```python
from build123d import *

# Parameters (mm, degrees)
SKETCH1_R           = 2.8575
BOSS_EXTRUDE1_DEPTH = 3.5052
CUT_EXTRUDE1_DEPTH  = 1.9558
SKETCH3_R           = 1.7145
BOSS_EXTRUDE2_DEPTH = 25.4


with BuildPart() as part:
    # Sketch1 → Boss-Extrude1 (new body)
    with BuildSketch(Plane(origin=(0, 0, 0), x_dir=(1, 0, 0), z_dir=(0, 1, 0))):
        Circle(SKETCH1_R)
    extrude(amount=BOSS_EXTRUDE1_DEPTH)

    # Sketch2 → Cut-Extrude1 (cut)
    with BuildSketch(Plane.XZ):
        Polygon((1.603951217, 0), (0.801975608, 1.3890625), (-0.801975608, 1.3890625), (-1.603951217, 0), (-0.801975608, -1.3890625), (0.801975608, -1.3890625), align=None)
    extrude(amount=-CUT_EXTRUDE1_DEPTH, mode=Mode.SUBTRACT)

    # Sketch3 → Boss-Extrude2 (add)
    with BuildSketch(Plane(origin=(0, 3.5052, 0), x_dir=(1, 0, 0), z_dir=(0, 1, 0))):
        Circle(SKETCH3_R)
    extrude(amount=BOSS_EXTRUDE2_DEPTH)


solid = part.part
```
Check sheet for the modelled part. Datum: model origin and axes. Units: mm. A direction names the side the tool comes from. Round coordinates to 2 decimals unless told otherwise and drop trailing zeros. Order: outer loops, then holes, each group sorted by start corner. A loop starts at its lowest first (then second) coordinate and runs counter-clockwise, first axis right, second up. Notation, with made-up numbers: (15.25, 77) -> (42.25, 77) arc R20 cw to (42.25, 104) -> close; hole circle Ø6 at (33, 8.25). An arc over 180 degrees is marked (long way). Use CSV: the item, a comma, the result in double quotes.
(1) Depth check by flat-ended pin: pin 1 (2 mm diameter, centred on y = 21, z = 1.5, fed in from -X); pin 2 (2 mm diameter, centred on y = 3, z = 2, fed in from -X); pin 3 (2 mm diameter, centred on y = 11, z = -2, fed in from -X); pin 4 (2 mm diameter, centred on x = 0.5, z = 0, fed in from -Y). Enter the tip coordinate at first touch or a pass-through.
Worked out:
pin 1,"x = -1.64"
pin 2,"x = -2.68"
pin 3,"x = -1.39"
pin 4,"y = 0"
(2) Cross-section at A-A (x = 0). Record the boundary of the cut face in (y, z).
Worked out:
outline,"(0, -2.86) -> (3.51, -2.86) -> (3.51, -1.71) -> (28.91, -1.71) -> (28.91, 1.71) -> (3.51, 1.71) -> (3.51, 2.86) -> (0, 2.86) -> (0, 1.39) -> (1.96, 1.39) -> (1.96, -1.39) -> (0, -1.39) -> close"
(3) Cross-section at D-D (y = 21.5). Record the boundary of the cut face in (x, z), and give its area (3 significant figures).
Worked out:
outline,"circle Ø3.43 at (0, 0)"
area,"9.23 mm²"
(4) Tool access check on faces 4 (the face through (0, 3.505, 2)), 5 (the face through (0, 1, 1.389)), 6 (the face through (1.2, 0, 1.2)). Record the directions out of +Z, -Z, +X, -X, +Y, -Y that give a thin tool (end or side, any length) a straight path to the whole face; none if there is none.
Worked out:
face 4,"+Y"
face 5,"-Y"
face 6,"+Z, -Z, +X, -X, -Y"
(5) Cross-section at C-C (y = 2.5). Record the boundary of the cut face in (x, z) (1 decimal).
Worked out:
outline,"circle Ø5.7 at (0, 0)"
(6) Material ranges on line 1 along Y through (x, z) = (-1.65, 1.25); line 2 along Y through (x, z) = (-0.6, -0.3); line 3 along X through (y, z) = (26.25, 1), recorded low to high. Write a range as from..to.
Worked out:
line 1,"0..3.51"
line 2,"1.96..28.91"
line 3,"-1.39..1.39"
(7) Draft check along X on faces 1 (the face through (2.726, 1.728, -0.858)), 2 (the face through (0, 1.956, 0)), 3 (the face through (0, 28.905, 0)). Enter one of: pulls with the +X half, pulls with the -X half, needs draft (parallel to the pull), parting line crosses it, or undercut.
Worked out:
face 1,"parting line crosses it"
face 2,"undercut"
face 3,"needs draft"
(8) Cross-section at B-B (z = 0.25). Record the boundary of the cut face in (x, y), and give its area (3 significant figures).
Worked out:
outline,"(-2.85, 0) -> (-1.46, 0) -> (-1.46, 1.96) -> (1.46, 1.96) -> (1.46, 0) -> (2.85, 0) -> (2.85, 3.51) -> (1.7, 3.51) -> (1.7, 28.91) -> (-1.7, 28.91) -> (-1.7, 3.51) -> (-2.85, 3.51) -> close"
area,"100 mm²"
